Geometry: final body of the model. Coordinates: model frame, mm. Coordinates: 2 decimals unless noted, no trailing zeros. Order: outer loops, then holes, each group sorted by start corner. A loop starts at its lowest first (then second) coordinate and runs counter-clockwise, first axis right, second up. Notation, with made-up numbers: (32.5, -21) - (57.5, -21) arc R15 cw to (57.5, -16) - close; hole circle Ø8 at (11.25, -16). An arc over 180 degrees is marked (long way). Use a Markdown table: item, result. Add a question column.
```python
from build123d import *

# Parameters (mm, degrees)
BOSS_EXTRUDE1_DEPTH = 2.3622
SKETCH2_R           = 2
SKETCH2_W           = 156
SKETCH2_H           = 91
CUT_EXTRUDE1_DEPTH  = 119.672908335


with BuildPart() as part:
    # Sketch1 → Boss-Extrude1 (new body)
    with BuildSketch(Plane(origin=(0, 0, 0), x_dir=(1, 0, 0), z_dir=(0, 1, 0))):
        Polygon((-93.522777066, 66.883834733), (-73.522777066, 66.883834733), (-73.522777066, 69.883834733), (-53.522777066, 69.883834733), (-53.522777066, 66.883834733), (41.752822934, 66.883834733), (41.752822934, 69.883834733), (61.752822934, 69.883834733), (61.752822934, 66.883834733), (81.752822934, 66.883834733), (81.752822934, 49.193834733), (84.115022934, 49.193834733), (84.115022934, 29.193834733), (81.752822934, 29.193834733), (81.752822934, -15.806165267), (84.115022934, -15.806165267), (84.115022934, -35.806165267), (81.752822934, -35.806165267), (81.752822934, -55.806165267), (-93.522777066, -55.806165267), (-93.522777066, -35.806165267), (-95.884977066, -35.806165267), (-95.884977066, -15.806165267), (-93.522777066, -15.806165267), (-93.522777066, 29.193834733), (-95.884977066, 29.193834733), (-95.884977066, 49.193834733), (-93.522777066, 49.193834733), align=None)
    extrude(amount=BOSS_EXTRUDE1_DEPTH)

    # Sketch2 → Cut-Extrude1 (cut, through all)
    with BuildSketch(Plane(origin=(0, 2.3622, 0), x_dir=(1, 0, 0), z_dir=(0, 1, 0))):
        with Locations(Location((-63.384977066, 58.883834733, 0), (0, 0, 270))):
            Circle(SKETCH2_R)
        with Locations(Location((51.615022934, 58.883834733, 0), (0, 0, 270))):
            Circle(SKETCH2_R)
        with Locations(Location((-63.384977066, -46.116165267, 0), (0, 0, 270))):
            Circle(SKETCH2_R)
        with Locations(Location((51.615022934, -46.116165267, 0), (0, 0, 270))):
            Circle(SKETCH2_R)
        with Locations((-5.884977066, 6.383834733)):
            Rectangle(SKETCH2_W, SKETCH2_H)
    extrude(amount=-CUT_EXTRUDE1_DEPTH, mode=Mode.SUBTRACT)


solid = part.part
```
1) Section query D-D (y = 1.7). Give the number of separate pieces and of enclosed holes in the cut face, and give its area (3 significant figures).
2) Section query C-C (z = -55). Return the cut outline in (x, y).
3) Section query B-B (z = 12). Return the cut outline in (x, y).
4) Line query: line 1 (X direction, y = 0.4, z = -59); line 2 (Z direction, x = 61.5, y = 1.6); line 3 (X direction, y = 0.35, z = 21). Output: solid intervals per line, ascending. Write a range as from..to.
5) Section query A-A (x = 23.5). Return the cut outline in (y, z).
6) First-contact query: pin 1 (0.7 mm diameter, centred on y = 1, z = -68, fed in from -X); pin 2 (1.2 mm diameter, centred on y = 1, z = 41.5, fed in from +X); pin 3 (1.2 mm diameter, centred on x = -6, y = 1.5, fed in from -Z); pin 4 (3.5 mm diameter, centred on x = 51.62, z = -58.88, fed in from -Y). Flat tips, straight axial feed; report the tip coordinate or a pass-through.
7) Draft query along X for faces 1 (the flat face through (-5, 2.362, 48)), 2 (the cylindrical face through (50.4, 1.2, 44.53)). Return one class per face: released by +X, released by -X, zero draft, split by the parting line, or undercut.
From the geometry:
| question | item | result |
|---|---|---|
| 1 | separate pieces | 1 |
| 1 | enclosed holes | 5 |
| 1 | area | 7,570 mm^2 |
| 2 | outline | (-93.52, 0) - (81.75, 0) - (81.75, 2.36) - (-93.52, 2.36) - close |
| 3 | outline | (-93.52, 0) - (-83.88, 0) - (-83.88, 2.36) - (-93.52, 2.36) - close; (72.12, 0) - (81.75, 0) - (81.75, 2.36) - (72.12, 2.36) - close |
| 4 | line 1 | x = -93.52..-65.38, -61.39..49.62, 53.61..81.75 |
| 4 | line 2 | z = -69.88..-51.88, 39.12..55.81 |
| 4 | line 3 | x = -95.88..-83.88, 72.12..84.12 |
| 5 | outline | (0, -66.88) - (2.36, -66.88) - (2.36, -51.88) - (0, -51.88) - close; (0, 39.12) - (2.36, 39.12) - (2.36, 55.81) - (0, 55.81) - close |
| 6 | pin 1 | stops at x = -73.52 |
| 6 | pin 2 | stops at x = 81.75 |
| 6 | pin 3 | stops at z = -66.88 |
| 6 | pin 4 | passes through |
| 7 | face 1 | zero draft |
| 7 | face 2 | undercut |
